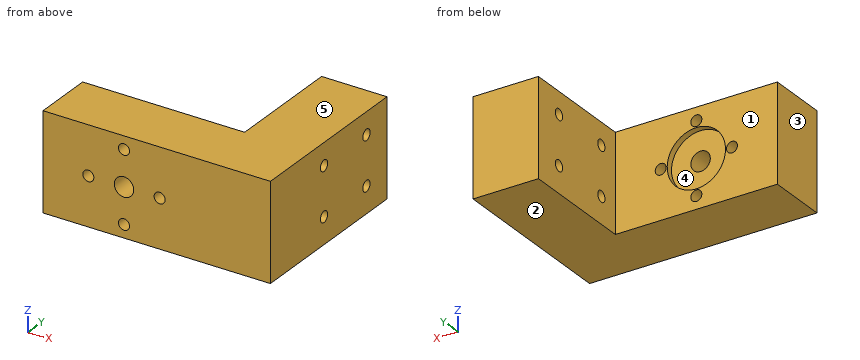
```python
from build123d import *

# Parameters (mm, degrees)
BOSS_EXTRUDE1_DEPTH = 30
SKETCH2_R           = 9
CUT_EXTRUDE1_DEPTH  = 2
SKETCH4_R           = 1.7
SKETCH4_R_2         = 3
CUT_EXTRUDE2_DEPTH  = 85.524115494
SKETCH5_R           = 1.7
CUT_EXTRUDE3_DEPTH  = 95.083133983


with BuildPart() as part:
    # Sketch1 → Boss-Extrude1 (new body)
    with BuildSketch(Plane.XY):
        Polygon((0, 0), (0, 18.7), (50, 18.7), (50, 55), (70.19, 55), (70.19, 0), align=None)
    extrude(amount=-BOSS_EXTRUDE1_DEPTH)

    # Sketch2 → Cut-Extrude1 (cut)
    with BuildSketch(Plane(origin=(0, 18.7, 0), x_dir=(1, 0, 0), z_dir=(0, 1, 0))):
        with Locations(Location((25, 15, 0), (0, 0, 270))):
            Circle(SKETCH2_R)
    extrude(amount=-CUT_EXTRUDE1_DEPTH, mode=Mode.SUBTRACT)

    # Sketch4 → Cut-Extrude2 (cut, through all)
    with BuildSketch(Plane(origin=(0, 18.7, 0), x_dir=(1, 0, 0), z_dir=(0, 1, 0))):
        with Locations(Location((25, 26, 0), (0, 0, 270))):
            Circle(SKETCH4_R)
        with Locations(Location((36, 15, 0), (0, 0, 270))):
            Circle(SKETCH4_R)
        with Locations(Location((25, 4, 0), (0, 0, 270))):
            Circle(SKETCH4_R)
        with Locations(Location((14, 15, 0), (0, 0, 270))):
            Circle(SKETCH4_R)
        with Locations(Location((25, 15, 0), (0, 0, 270))):
            Circle(SKETCH4_R_2)
    extrude(amount=-CUT_EXTRUDE2_DEPTH, mode=Mode.SUBTRACT)

    # Sketch5 → Cut-Extrude3 (cut, through all)
    with BuildSketch(Plane(origin=(70.19, 0, 0), x_dir=(0, 0, -1), z_dir=(1, 0, 0))):
        with Locations(Location((6.810503995, 45.303971798, 0), (0, 0, 90))):
            Circle(SKETCH5_R)
        with Locations(Location((6.810503995, 25.303971798, 0), (0, 0, 90))):
            Circle(SKETCH5_R)
        with Locations(Location((21.810503995, 45.303971798, 0), (0, 0, 90))):
            Circle(SKETCH5_R)
        with Locations(Location((21.810503995, 25.303971798, 0), (0, 0, 90))):
            Circle(SKETCH5_R)
    extrude(amount=-CUT_EXTRUDE3_DEPTH, mode=Mode.SUBTRACT)


solid = part.part
```
Model file for the job. Use its own axes, mm. Face numbers are marked on the shaded views. A direction names the side the tool comes from. Coordinates: 2 decimals unless noted, no trailing zeros. Loops run counter-clockwise (first coordinate to the right, second up) from the corner with the lowest first, then second, coordinate; pieces in that order, holes last. Notation, with made-up numbers: M 47.25,-29 L 91.25,-29 A17 ccw 91.25,-22 Z; hole C 13,8.5 d5. An arc over 180 degrees is marked long. Use CSV: the item, a comma, the result in double quotes. Start each with the question number.
1. Probe probe 1 along X at (y, z) = (6, -15); probe 2 along Y at (x, z) = (54, -23.25); probe 3 along Y at (x, z) = (9.5, -13.75). List the from-to ranges inside material, lowest first. Write a range as [from, to].
2. Band-saw the part on A-A, the plane z = -4. List the corners of the cut face in (x, y), then the cut area to 3 significant figures.
3. Flat gauge pins, fed straight in: pin 1 (9 mm diameter, centred on x = 24.5, z = -13.5, fed in from +Y); pin 2 (9 mm diameter, centred on y = 30, z = -20.5, fed in from -X). Where does each tip first touch, or does it go through?
4. Tool access for the marked faces 1 and 2: list every direction of +Z, -Z, +X, -X, +Y, -Y with a clear straight run to the whole face (end or side of a thin tool).
5. Band-saw the part on C-C, the plane y = 6. List the corners of the cut face in (x, z).
6. Two-plate mould, pull along X, no slides. Class the marked faces 3, 4 and 5: pulls with the +X half, pulls with the -X half, needs draft (parallel to the pull), parting line crosses it, or undercut.
7. Band-saw the part on D-D, the plane x = 14. List the corners of the cut face in (y, z).
8. Band-saw the part on B-B, the plane x = 25. List the corners of the cut face in (y, z).
Entries:
1,probe 1,"x = [0, 12.3], [15.7, 22], [28, 34.3], [37.7, 70.19]"
1,probe 2,"y = [0, 24.4], [26.21, 44.4], [46.21, 55]"
1,probe 3,"y = [0, 18.7]"
2,outline,"M 0,0 L 23.3,0 L 23.3,18.7 L 0,18.7 Z; M 26.7,0 L 70.19,0 L 70.19,55 L 50,55 L 50,18.7 L 26.7,18.7 Z"
2,area,"1,980 mm2"
3,pin 1,"stops at y = 16.7"
3,pin 2,"stops at x = 50"
4,face 1,"+Z, -Z, -X, +Y"
4,face 2,"-Z, +X, -X, +Y, -Y"
5,outline,"M 0,-30 L 70.19,-30 L 70.19,0 L 0,0 Z; hole C 14,-15 d3.4; hole C 25,-15 d6; hole C 25,-26 d3.4; hole C 25,-4 d3.4; hole C 36,-15 d3.4"
6,face 3,"pulls with the -X half"
6,face 4,"undercut"
6,face 5,"needs draft"
7,outline,"M 0,-30 L 18.7,-30 L 18.7,-16.7 L 0,-16.7 Z; M 0,-13.3 L 18.7,-13.3 L 18.7,0 L 0,0 Z"
8,outline,"M 0,-30 L 18.7,-30 L 18.7,-27.7 L 0,-27.7 Z; M 0,-24.3 L 18.7,-24.3 L 18.7,-24 L 16.7,-24 L 16.7,-18 L 0,-18 Z; M 0,-12 L 16.7,-12 L 16.7,-6 L 18.7,-6 L 18.7,-5.7 L 0,-5.7 Z; M 0,-2.3 L 18.7,-2.3 L 18.7,0 L 0,0 Z"
